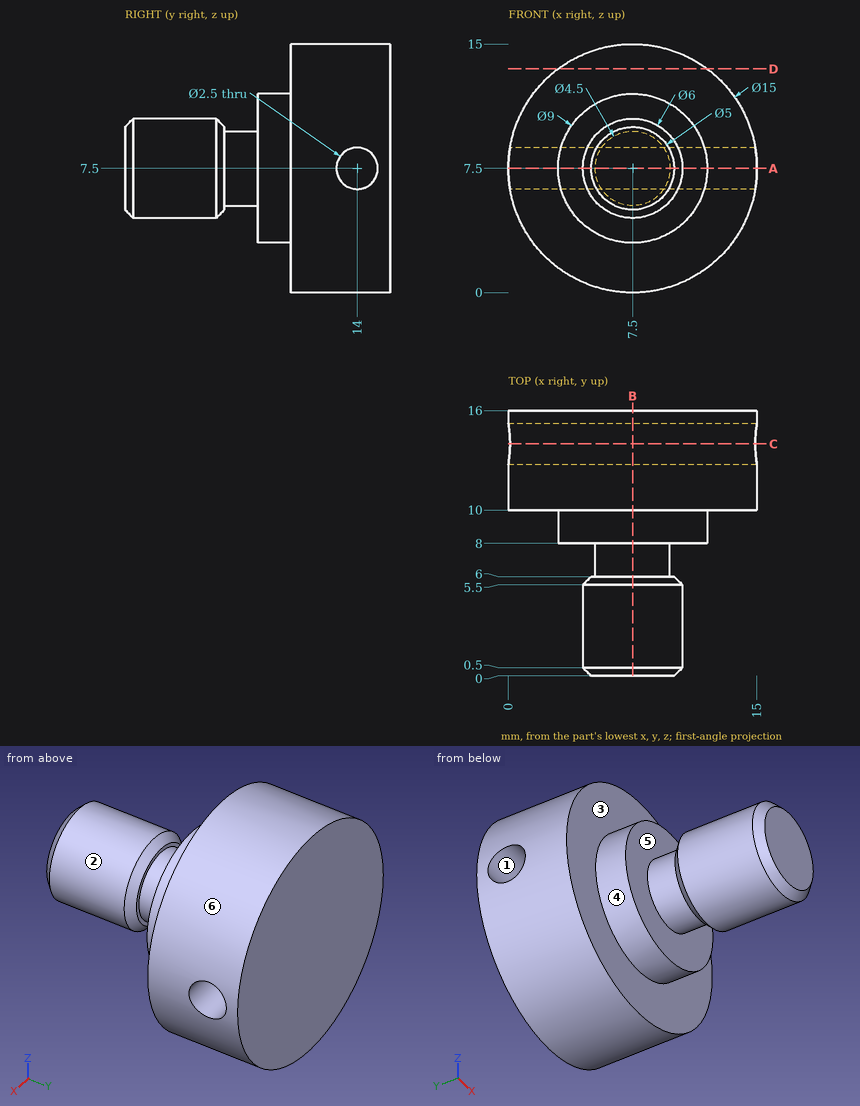
Check sheet for the drawn part. Datum: minimum x, y, z corner. Units: mm. A direction names the side the tool comes from. Coordinates: 2 decimals unless noted, no trailing zeros. Order: outer loops, then holes, each group sorted by start corner. A loop starts at its lowest first (then second) coordinate and runs counter-clockwise, first axis right, second up. Notation, with made-up numbers: (31, -16) -> (85, -16) arc R13 cw to (85, 9) -> close; hole circle Ø8 at (7, 33.5). An arc over 180 degrees is marked (long way). Use a Markdown table: item, result. Add a question column.
1. Mould release check, pull along Z, two halves, no side actions. Record for the marked faces 1, 2 and 3: pulls with the +Z half, pulls with the -Z half, needs draft (parallel to the pull), parting line crosses it, or undercut.
2. Cross-section at B-B (x = 7.5). Enter the section's corners in (y, z).
3. Cross-section at D-D (z = 13.5). Enter the section's corners in (x, y), and give its area (3 significant figures).
4. Material ranges on L1, parallel to Y at x = 9.25, z = 9; L2, parallel to Y at x = 11.5, z = 2.5; L3, parallel to Y at x = 4, z = 5.5, recorded low to high.
5. Cross-section at A-A (z = 7.5). Enter the section's corners in (x, y).
6. Cross-section at C-C (y = 14). Enter the section's corners in (x, z).
7. Go/stop test with flat-tipped pins: pin 1 Ø1 at (y, z) = (9, 13) entering from +X; pin 2 Ø3 at (y, z) = (10, 11.5) entering from -X; pin 3 Ø4 at (y, z) = (4, 4.5) entering from +X. Record where each tip stops, or that it passes through.
8. Set-up check for the marked faces 4, 5 and 6: record each of +Z, -Z, +X, -X, +Y, -Y from which the full face is reachable in a straight line by a thin tool's end or side.
Filled sheet:
| question | item | result |
|---|---|---|
| 1 | face 1 | undercut |
| 1 | face 2 | parting line crosses it |
| 1 | face 3 | needs draft |
| 2 | outline | (0, 5) -> (0.5, 4.5) -> (5.5, 4.5) -> (6, 5) -> (6, 5.25) -> (8, 5.25) -> (8, 3) -> (10, 3) -> (10, 0) -> (16, 0) -> (16, 15) -> (10, 15) -> (10, 12) -> (8, 12) -> (8, 9.75) -> (6, 9.75) -> (6, 10) -> (5.5, 10.5) -> (0.5, 10.5) -> (0, 10) -> close; hole circle Ø2.5 at (14, 7.5) |
| 3 | outline | (3, 10) -> (12, 10) -> (12, 16) -> (3, 16) -> close |
| 3 | area | 54.0 mm2 |
| 4 | L1 | 0 to 6, 8 to 16 |
| 4 | L2 | 10 to 16 |
| 4 | L3 | 8 to 16 |
| 5 | outline | (0, 10) -> (3, 10) -> (3, 8) -> (5.25, 8) -> (5.25, 6) -> (5, 6) -> (4.5, 5.5) -> (4.5, 0.5) -> (5, 0) -> (10, 0) -> (10.5, 0.5) -> (10.5, 5.5) -> (10, 6) -> (9.75, 6) -> (9.75, 8) -> (12, 8) -> (12, 10) -> (15, 10) -> (15, 12.75) -> (0, 12.75) -> close; (0, 15.25) -> (15, 15.25) -> (15, 16) -> (0, 16) -> close |
| 6 | outline | (0.1, 6.25) arc R7.5 ccw to (14.9, 6.25) -> close; (0.1, 8.75) -> (14.9, 8.75) arc R7.5 ccw to start |
| 7 | pin 1 | through |
| 7 | pin 2 | x = 0.43 |
| 7 | pin 3 | x = 10.33 |
| 8 | face 4 | -Y |
| 8 | face 5 | none |
| 8 | face 6 | +Y, -Y |
